Print and shaded views of the part. All mm, measured from the part's lowest x, y and z. A direction names the side the tool comes from. Coordinates: 2 decimals unless noted, no trailing zeros. Order: outer loops, then holes, each group sorted by start corner. A loop starts at its lowest first (then second) coordinate and runs counter-clockwise, first axis right, second up. Notation, with made-up numbers: M -9,-25.75 L -2,-25.75 A18 cw -2,4.25 Z; hole C 79,27.5 d5. An arc over 180 degrees is marked long. Return JSON: item names as keys, results as strings.
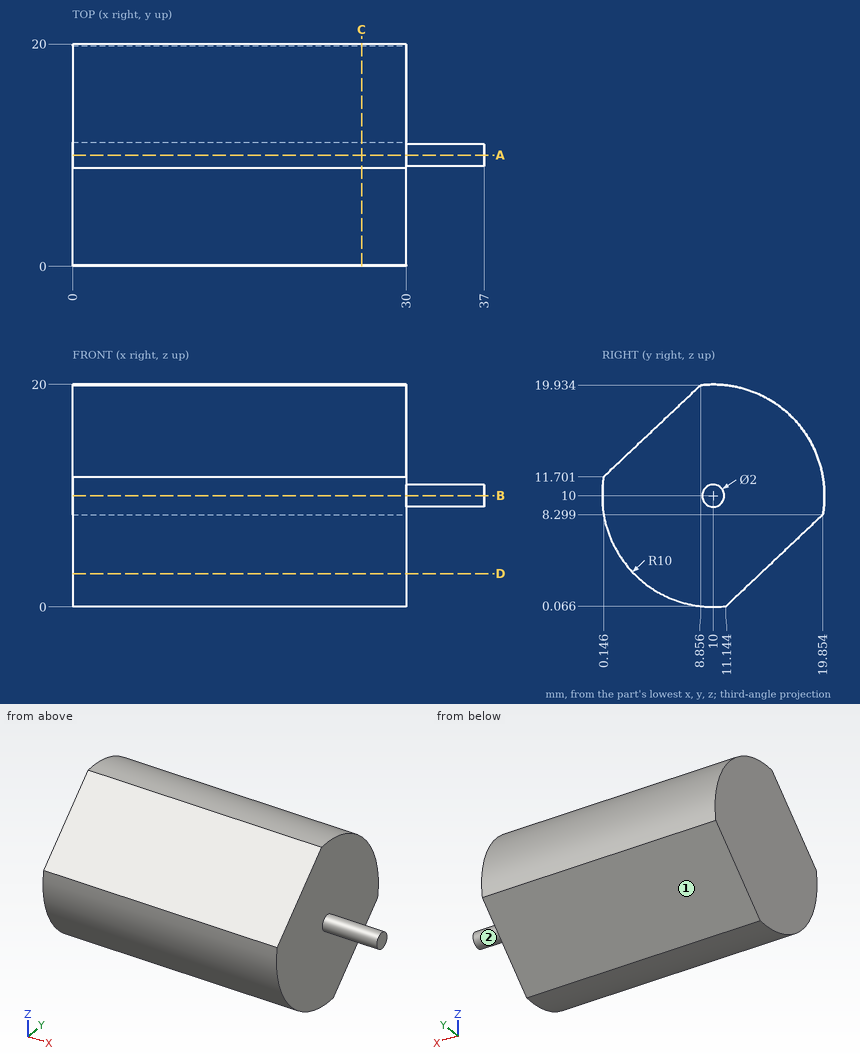
Item 1: Drop flat-ended pins along their axis: pin 1 Ø10 at (x, z) = (26, 4.5) entering from -Y; pin 2 Ø5 at (y, z) = (7.5, 17.5) entering from +X; pin 3 Ø6 at (x, y) = (9.5, 6) entering from -Z. Give the stop position or say it passes through.
Check result:
{"pin 1": "stops at y = 0.01", "pin 2": "stops at x = 30", "pin 3": "stops at z = 0.05"}
Item 2: Wall check: line 1 (X direction, y = 6, z = 1.75); line 2 (Z direction, x = 5.5, y = 9.75); line 3 (Z direction, x = 4.5, y = 5.25) (1 decimal). Give the ranges that are in metal, low to high.
Check result:
{"line 1": "x = 0 to 30", "line 2": "z = 0 to 20", "line 3": "z = 1.2 to 16.5"}
Item 3: 3-axis set-ups, long thin cutter, end or side, ignore diameter. For the marked faces 1 and 2: which of +Z, -Z, +X, -X, +Y, -Y reach the whole face in a straight line?
Check result:
{"face 1": "-Z, +X, -X, +Y", "face 2": "+X"}
Item 4: Saw through at D-D (z = 3). Write the cut outline in (x, y).
Check result:
{"outline": "M 0,2.86 L 30,2.86 L 30,14.25 L 0,14.25 Z"}
Item 5: Saw through at A-A (y = 10). Write the cut outline in (x, z).
Check result:
{"outline": "M 0,0 L 30,0 L 30,9 L 37,9 L 37,11 L 30,11 L 30,20 L 0,20 Z"}
Item 6: Saw through at C-C (x = 26). Write the cut outline in (y, z) (1 decimal), and give its area (3 significant figures).
Check result:
{"outline": "M 0.1,11.7 A10 ccw 11.1,0.1 L 19.9,8.3 A10 ccw 8.9,19.9 Z", "area": "282 mm2"}
